Can you work these out from the drawing? Everything is in mm from the part's minimum corner. A direction names the side the tool comes from. Round coordinates to 2 decimals unless told otherwise and drop trailing zeros. Loops run counter-clockwise (first coordinate to the right, second up) from the corner with the lowest first, then second, coordinate; pieces in that order, holes last. Notation, with made-up numbers: (70, 60.5) -> (111, 60.5) arc R23 cw to (111, 95.5) -> close; hole circle Ø9 at (33, 50.5). An arc over 180 degrees is marked (long way). Answer as a JSON object with one key per item and string values.
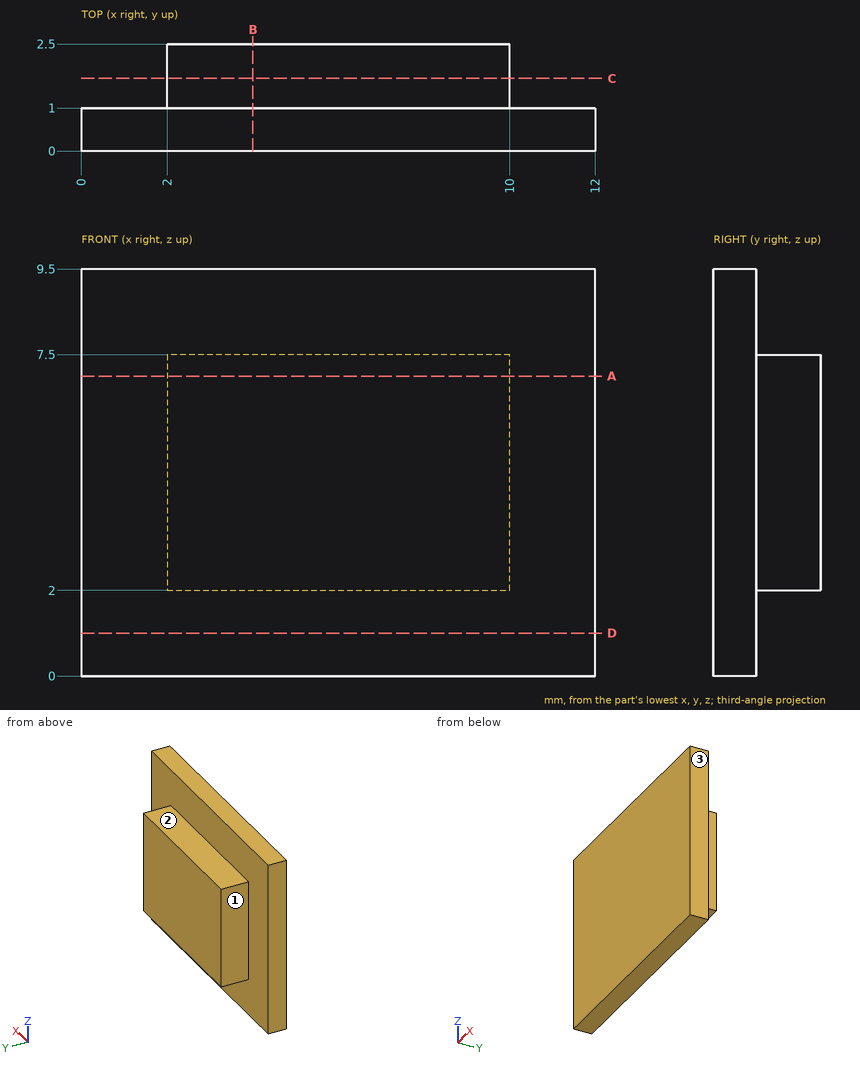
Q1. If I drill on L1, parallel to X at y = 2.05, z = 6; L2, parallel to Y at x = 2.75, z = 1.75; L3, parallel to Z at x = 3.75, y = 2, over which ranges is the centre line in solid material (lowest first)? Write a range as [from, to].
Determined:
{"L1": "[2, 10]", "L2": "[0, 1]", "L3": "[2, 7.5]"}
Q2. I want a section at B-B, the plane x = 4. Write out the boundary of the cut face in (y, z).
Determined:
{"outline": "(0, 0) -> (1, 0) -> (1, 2) -> (2.5, 2) -> (2.5, 7.5) -> (1, 7.5) -> (1, 9.5) -> (0, 9.5) -> close"}
Q3. I want a section at A-A, the plane z = 7. Write out the boundary of the cut face in (x, y), then the cut area to 3 significant figures.
Determined:
{"outline": "(0, 0) -> (12, 0) -> (12, 1) -> (10, 1) -> (10, 2.5) -> (2, 2.5) -> (2, 1) -> (0, 1) -> close", "area": "24.0 mm²"}
Q4. I want a section at C-C, the plane y = 1.7. Write out the boundary of the cut face in (x, z).
Determined:
{"outline": "(2, 2) -> (10, 2) -> (10, 7.5) -> (2, 7.5) -> close"}
Q5. I want a section at D-D, the plane z = 1. Write out the boundary of the cut face in (x, y).
Determined:
{"outline": "(0, 0) -> (12, 0) -> (12, 1) -> (0, 1) -> close"}
Q6. I'm going to push flat-ended pins straight in: pin 1 (0.8 mm diameter, centred on x = 6, y = 2, fed in from -Z); pin 2 (1.2 mm diameter, centred on y = 2, z = 5, fed in from -X); pin 3 (1.5 mm diameter, centred on x = 2, z = 1, fed in from +Y). Where does each tip first touch, or does it pass through?
Determined:
{"pin 1": "z = 2", "pin 2": "x = 2", "pin 3": "y = 1"}
Q7. On a 3-axis mill with a long thin cutter (end or side, diameter ignored), from which of +Z, -Z, +X, -X, +Y, -Y can I reach the whole of each face in a straight line? I mean the marked faces 1, 2 and 3. Say none if no direction works.
Determined:
{"face 1": "+Z, -Z, -X, +Y", "face 2": "+Z, +X, -X, +Y", "face 3": "+Z, -Z, +X, +Y, -Y"}
